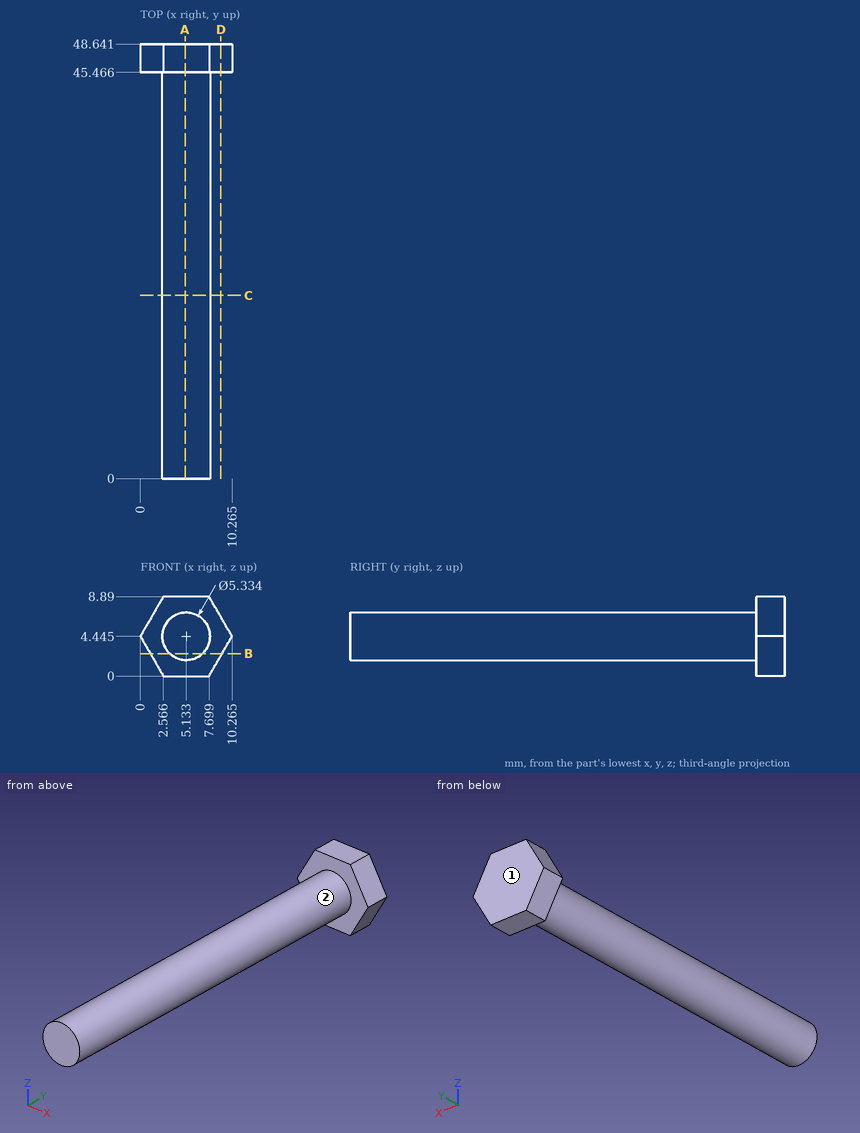
Could you check a few things on this drawing? It's one solid part, dimensions in mm from its lowest x, y, z. A direction names the side the tool comes from. Coordinates: 2 decimals unless noted, no trailing zeros. Order: outer loops, then holes, each group sorted by start corner. A loop starts at its lowest first (then second) coordinate and runs counter-clockwise, first axis right, second up.
1. If we section it at D-D (x = 9): Please give me the cut outline in (y, z), then the cut area to 3 significant figures.
2. If we section it at A-A (x = 5): Please give me the cut outline in (y, z).
3. I'm going to push flat-ended pins straight in: pin 1 (3 mm diameter, centred on y = 43.5, z = 1.5, fed in from +X) (1 decimal); pin 2 (1.5 mm diameter, centred on x = 4, y = 30.5, fed in from +Z); pin 3 (4 mm diameter, centred on y = 18.5, z = 5.5, fed in from +X). Where does each tip first touch, or does it pass through?
4. If we section it at B-B (z = 2.5): Please give me the cut outline in (x, y).
5. I need wall thicknesses on line 1 (Y direction, x = 8.5, z = 2); line 2 (X direction, y = 23, z = 3.5); line 3 (X direction, y = 30.5, z = 2.75) (1 decimal). Which ranges of each line are inside material? Lowest first, please.
6. For the marked faces 1 and 2, which set-ups out of +Z, -Z, +X, -X, +Y, -Y let a thin tool reach every point of the face, with its end or its side?
7. If we section it at C-C (y = 20.5): Please give me the cut outline in (x, z) (1 decimal).
Entries:
1. outline: (45.47, 2.25) - (48.64, 2.25) - (48.64, 6.64) - (45.47, 6.64) - close
1. area: 13.9 mm2
2. outline: (0, 1.78) - (45.47, 1.78) - (45.47, 0) - (48.64, 0) - (48.64, 8.89) - (45.47, 8.89) - (45.47, 7.11) - (0, 7.11) - close
3. pin 1: stops at x = 7.4
3. pin 2: stops at z = 7.08
3. pin 3: stops at x = 7.8
4. outline: (1.12, 45.47) - (3.31, 45.47) - (3.31, 0) - (6.96, 0) - (6.96, 45.47) - (9.14, 45.47) - (9.14, 48.64) - (1.12, 48.64) - close
5. line 1: y = 45.47 to 48.64
5. line 2: x = 2.64 to 7.63
5. line 3: x = 3.1 to 7.2
6. face 1: +Z, -Z, +X, -X, +Y
6. face 2: -Y
7. outline: circle Ø5.3 at (5.1, 4.4)
